For this review, take the finished solid that the model builds, in its own axes (mm). Round coordinates to 2 decimals unless told otherwise and drop trailing zeros. Loops run counter-clockwise (first coordinate to the right, second up) from the corner with the lowest first, then second, coordinate; pieces in that order, holes last.
1. Consider section D-D on z = 7. State the section outline as (x, y) points.
2. Draft analysis for pull direction X (two halves, no side actions). For faces 1 (the flat face through (18, 26, 4)), 2 (the cylindrical face through (13.63, 18.51, 3.94)), 3 (the flat face through (11, 26, 0)), state which applies: released by +X, released by -X, zero draft, split by the parting line, or undercut.
3. Consider section C-C on x = 15.25. State the section outline as (y, z) points, then the cut area to 3 significant figures.
4. To check wall thickness, follow line 1 along Y through (x, z) = (-15.25, 2); line 2 along X through (y, z) = (22, 3.75); line 3 along X through (y, z) = (46, 4.25). State the ranges of each line that lie inside material, in increasing order.
5. Clearance check with flat-ended pins moving along their axes: pin 1 Ø1 at (x, z) = (1, 6.5) entering from -Y; pin 2 Ø3 at (x, y) = (15.25, 5) entering from +Z. State where each tip first meets the part, or that it passes through.
6. Consider section A-A on y = 48.5. State the section outline as (x, z) points, then the cut area to 3 significant figures.
7. Consider section B-B on z = 2. State the section outline as (x, y) points.
from build123d import *

# Parameters (mm, degrees)
F0_W     = 36
F0_H     = 52
F1_DEPTH = 8
F3_D     = 3.4
F5_DEPTH = 52.001


with BuildPart() as f1:
    # F0 (on Top) → F1 (new body)
    with BuildSketch(Plane.XY):
        with Locations((0, 26)):
            Rectangle(F0_W, F0_H)
    extrude(amount=F1_DEPTH)

    # F3 (through all)
    with Locations(Plane.XY.offset(8)):
        with Locations((15.25, 48.5), (15.25, 5), (-15.25, 18), (-15.25, 48.5), (15.25, 18), (-15.25, 5)):
            Hole(F3_D / 2)

    # F4 (on face) → F5 (cut, through all)
    with BuildSketch(Plane.XZ):
        with BuildLine():
            ThreePointArc((-5, 0), (0, -5), (5, 0))
            Line((5, 0), (-5, 0))
        make_face()
        with BuildLine():
            Line((-5, 0), (5, 0))
            ThreePointArc((5, 0), (0, 5), (-5, 0))
        make_face()
    extrude(amount=-F5_DEPTH, mode=Mode.SUBTRACT)


solid = f1.part
Resolved:
1. outline: (-18, 0) - (18, 0) - (18, 52) - (-18, 52) - close; hole circle Ø3.4 at (-15.25, 5); hole circle Ø3.4 at (-15.25, 18); hole circle Ø3.4 at (-15.25, 48.5); hole circle Ø3.4 at (15.25, 5); hole circle Ø3.4 at (15.25, 18); hole circle Ø3.4 at (15.25, 48.5)
2. face 1: released by +X
2. face 2: undercut
2. face 3: zero draft
3. outline: (0, 0) - (3.3, 0) - (3.3, 8) - (0, 8) - close; (6.7, 0) - (16.3, 0) - (16.3, 8) - (6.7, 8) - close; (19.7, 0) - (46.8, 0) - (46.8, 8) - (19.7, 8) - close; (50.2, 0) - (52, 0) - (52, 8) - (50.2, 8) - close
3. area: 334 mm2
4. line 1: y = 0 to 3.3, 6.7 to 16.3, 19.7 to 46.8, 50.2 to 52
4. line 2: x = -18 to -3.31, 3.31 to 18
4. line 3: x = -18 to -2.63, 2.63 to 18
5. pin 1: stops at y = 0
5. pin 2: passes through
6. outline: (-18, 0) - (-16.95, 0) - (-16.95, 8) - (-18, 8) - close; (-13.55, 0) - (-5, 0) arc R5 cw to (5, 0) - (13.55, 0) - (13.55, 8) - (-13.55, 8) - close; (16.95, 0) - (18, 0) - (18, 8) - (16.95, 8) - close
6. area: 194 mm2
7. outline: (-18, 0) - (-4.58, 0) - (-4.58, 52) - (-18, 52) - close; (4.58, 0) - (18, 0) - (18, 52) - (4.58, 52) - close; hole circle Ø3.4 at (-15.25, 5); hole circle Ø3.4 at (-15.25, 18); hole circle Ø3.4 at (-15.25, 48.5); hole circle Ø3.4 at (15.25, 5); hole circle Ø3.4 at (15.25, 18); hole circle Ø3.4 at (15.25, 48.5)
